Read the model definition and answer for the solid it produces. Units are mm, in the model's axes. Face numbers are marked on the shaded views. Give positions to 0.01 mm unless a question says otherwise; leave off trailing zeros. Order: outer loops, then holes, each group sorted by start corner. A loop starts at its lowest first (then second) coordinate and runs counter-clockwise, first axis right, second up. Notation, with made-up numbers: (33.25, -15) - (89.25, -15) arc R16 cw to (89.25, -10) - close; hole circle Ø5 at (63.5, 56.25). An arc over 180 degrees is marked (long way). Return JSON: item names as keys, results as strings.
Autodesk Inventor part; units mm, degrees
ref_plane "Cross Section Plane" through (-7.7984, 1.2466, 0) normal (-0.1605, -0.987, 0) x (0, 0, 1)
ref_plane "Work Plane2" through (0.0562, -0.0303, 0) normal (-1, 0, 0) x (0, 0, 1)
ref_plane "Work Plane3" through (-0.3014, -71.6613, 0) normal (-0.0029, -1, 0) x (0, 0, 1)
sketch "Sketch Path" plane through (0, 0, 0) normal (0, 0, 1) x (1, 0, 0)
  arc A0 (7.9232, 1.1681) -> (-7.7984, 1.2466) centre (0.0562, -0.0303) ccw
  arc A1 (-19.1526, -68.5968) -> (18.5793, -68.7851) centre (-0.3014, -71.6613) ccw
  line L0 (-19.1526, -68.5968) -> (-7.7984, 1.2466)
  line L1 (7.9232, 1.1681) -> (18.5793, -68.7851)
ref_plane "Cross Section Plane" through (-7.7984, 1.2466, 0) normal (-0.1605, -0.987, 0) x (0, 0, 1)
ref_plane "Work Plane2" through (0.0562, -0.0303, 0) normal (-1, 0, 0) x (0, 0, 1)
ref_plane "Work Plane3" through (-0.3014, -71.6613, 0) normal (-0.0029, -1, 0) x (0, 0, 1)
sketch "Cross Section" plane through (-7.7984, 1.2466, 0) normal (-0.1605, -0.987, 0) x (0, 0, 1)
  line L0 (-2, 0.3) -> (2, 0.3)
  line L1 (2, 0.3) -> (2, -0.3)
  line L2 (2, -0.3) -> (-2, -0.3)
  line L3 (-2, -0.3) -> (-2, 0.3)
  line L4 (-2, 0) -> (2, 0) construction
  point P0 (0, 0)
  point P1 (0, 0)
  dimension "d0" = 4
  dimension "d4" = 0.3
  dimension "d5" = 0.3
sweep "Belt" add profiles "Cross Section" path "Sketch Path"
equation "\"d0\" = da_B"
equation "\"d4\" = da_a"
equation "\"d5\" = da_a2"
equation "\"da_B\" = 4"
equation "\"da_pb\" = 2.5"
equation "\"da_a\" = 0.3"
equation "\"da_S\" = 1.5"
equation "\"da_Beta\" = 20deg"
equation "\"da_Ht\" = 0.7"
equation "\"da_H\" = 1.3"
equation "\"da_a2\" = 0.3"
properties part number "Synchronous Belt" material "Rubber"
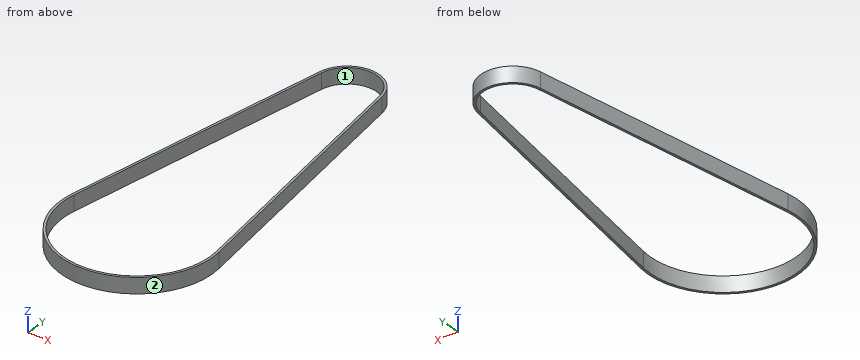
Q1. Determine the mould class of the marked faces 1 and 2 for opening direction X: released by +X, released by -X, zero draft, split by the parting line, or undercut.
Values:
{"face 1": "undercut", "face 2": "split by the parting line"}
Q2. A cutting plane is placed at B-B (y = -73.5). Write down the section's boundary in (x, z).
Values:
{"outline": "(-19.61, -2) - (-19.01, -2) - (-19.01, 2) - (-19.61, 2) - close; (18.41, -2) - (19.01, -2) - (19.01, 2) - (18.41, 2) - close"}
Q3. Consider L1, parallel to X at y = -80.5, z = 0.65; L2, parallel to Y at x = -0.5, z = 1; L3, parallel to X at y = -55, z = 1.85. Determine where each line is inside the solid, lowest interval first.
Values:
{"L1": "x = -17.57 to -16.89, 16.29 to 16.97", "L2": "y = -91.06 to -90.46, 7.61 to 8.21", "L3": "x = -17.25 to -16.64, 16.18 to 16.78"}
Q4. A cutting plane is placed at A-A (x = 5.5). Write down the section's boundary in (y, z), and give its area (3 significant figures).
Values:
{"outline": "(-90.17, -2) - (-89.54, -2) - (-89.54, 2) - (-90.17, 2) - close; (5.36, -2) - (6.18, -2) - (6.18, 2) - (5.36, 2) - close", "area": "5.81 mm²"}
Q5. A cutting plane is placed at C-C (z = 0.25). Write down the section's boundary in (x, y).
Values:
{"outline": "(-19.45, -68.55) arc R19.4 ccw (long way) to (18.88, -68.74) - (8.22, 1.21) arc R8.26 ccw to (-8.09, 1.29) - close; hole (-18.86, -68.64) arc R18.8 ccw (long way) to (18.28, -68.83) - (7.63, 1.12) arc R7.66 ccw to (-7.5, 1.2) - close"}
